from build123d import *

# Parameters (mm, degrees)
F0_W          = 76.2
F0_H          = 38.1
F1_DEPTH      = 12.7
F2_R          = 19.05
F3_DEPTH      = 19.05
F4_R          = 19.05
F5_DEPTH      = 19.05
F6_R          = 7.9375
F7_DEPTH      = 19.051
F7_DEPTH_BACK = 31.751
F9_START      = -6.35
F8_R          = 14.9225
F8_R_2        = 7.9375
F9_DEPTH      = 6.35


with BuildPart() as f1:
    # F0 (on Top) → F1 (new body)
    with BuildSketch(Plane.XY):
        with Locations((38.1, 19.05)):
            Rectangle(F0_W, F0_H)
    extrude(amount=F1_DEPTH)

    # F2 (on face) → F3 (join)
    with BuildSketch(Plane.XY.offset(12.7)):
        with Locations((38.1, 19.05)):
            Circle(F2_R)
    extrude(amount=F3_DEPTH)

    # F4 (on face) → F5 (join)
    with BuildSketch(Plane(origin=(0, 0, 0), x_dir=(1, 0, 0), z_dir=(0, 0, -1))):
        with Locations((38.1, -19.05)):
            Circle(F4_R)
    extrude(amount=F5_DEPTH)

    # F6 (on Top) → F7 (cut, two sides)
    with BuildSketch(Plane.XY) as f7_sk:
        with Locations((38.1, 19.05)):
            Circle(F6_R)
    extrude(amount=-F7_DEPTH, mode=Mode.SUBTRACT)
    extrude(f7_sk.sketch, amount=F7_DEPTH_BACK, mode=Mode.SUBTRACT)

    # F8 (on face) → F9 (cut)
    with BuildSketch(Plane.XY.offset(31.75).offset(F9_START)):
        with Locations((38.1, 19.05)):
            Circle(F8_R)
        with Locations((38.1, 19.05)):
            Circle(F8_R_2, mode=Mode.SUBTRACT)
    extrude(amount=-F9_DEPTH, mode=Mode.SUBTRACT)


solid = f1.part
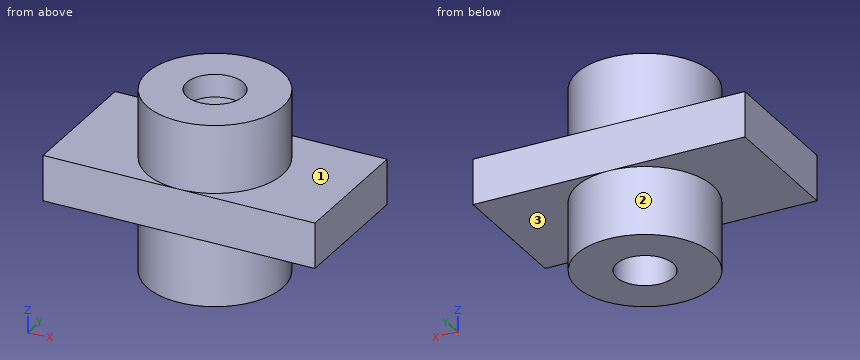
Part model, mm, in its own coordinate system. Face numbers are marked on the shaded views. A direction names the side the tool comes from. Coordinates: 2 decimals unless noted, no trailing zeros. Order: outer loops, then holes, each group sorted by start corner. A loop starts at its lowest first (then second) coordinate and runs counter-clockwise, first axis right, second up. Notation, with made-up numbers: (-0.75, 4.5) - (44.25, 4.5) arc R22 cw to (44.25, 22.5) - close; hole circle Ø8 at (88, 8.25). An arc over 180 degrees is marked (long way). Use CSV: the item, a comma, the result in double quotes.
Item 1: Saw through at A-A on y = 19.05. Give the cut face in (x, z).
Solved:
outline,"(0, 0) - (19.05, 0) - (19.05, -19.05) - (30.16, -19.05) - (30.16, 19.05) - (23.18, 19.05) - (23.18, 25.4) - (30.16, 25.4) - (30.16, 31.75) - (19.05, 31.75) - (19.05, 12.7) - (0, 12.7) - close; (46.04, -19.05) - (57.15, -19.05) - (57.15, 0) - (76.2, 0) - (76.2, 12.7) - (57.15, 12.7) - (57.15, 31.75) - (46.04, 31.75) - (46.04, 25.4) - (53.02, 25.4) - (53.02, 19.05) - (46.04, 19.05) - close"
Item 2: Saw through at C-C on x = 49. Give the cut face in (y, z), and give its area (3 significant figures).
Solved:
outline,"(0, 0) - (3.43, 0) - (3.43, -19.05) - (34.67, -19.05) - (34.67, 0) - (38.1, 0) - (38.1, 12.7) - (34.67, 12.7) - (34.67, 31.75) - (3.43, 31.75) - (3.43, 12.7) - (0, 12.7) - close; hole (8.86, 19.05) - (29.24, 19.05) - (29.24, 25.4) - (8.86, 25.4) - close"
area,"1,540 mm²"
Item 3: Probe probe 1 along Y at (x, z) = (38, 16.5); probe 2 along Y at (x, z) = (38.1, 21.25); probe 3 along Z at (x, y) = (50.5, 26.5). List the from-to ranges inside material, lowest first.
Solved:
probe 1,"y = 0 to 11.11, 26.99 to 38.1"
probe 2,"y = 0 to 4.13, 33.97 to 38.1"
probe 3,"z = -19.05 to 19.05, 25.4 to 31.75"
Item 4: Saw through at B-B on x = 36. Give the cut face in (y, z), and give its area (3 significant figures).
Solved:
outline,"(0, 0) - (0.12, 0) - (0.12, -19.05) - (11.4, -19.05) - (11.4, 19.05) - (4.28, 19.05) - (4.28, 25.4) - (11.4, 25.4) - (11.4, 31.75) - (0.12, 31.75) - (0.12, 12.7) - (0, 12.7) - close; (26.7, -19.05) - (37.98, -19.05) - (37.98, 0) - (38.1, 0) - (38.1, 12.7) - (37.98, 12.7) - (37.98, 31.75) - (26.7, 31.75) - (26.7, 25.4) - (33.82, 25.4) - (33.82, 19.05) - (26.7, 19.05) - close"
area,"1,060 mm²"
Item 5: Drop flat-ended pins along their axis: P1, Ø6, axis at y = 9.5, z = 15.5, coming from the -X side; P2, Ø1, axis at y = 28.5, z = -12.5, coming from the -X side; P3, Ø8, axis at y = 11, z = 21.5, coming from the +X side; P4, Ø3, axis at x = 63.5, y = 32, coming from the -Z side. Give the stop position or say it passes through.
Solved:
P1,"stops at x = 0"
P2,"stops at x = 21.28"
P3,"stops at x = 56.71"
P4,"stops at z = 0"
Item 6: 3-axis set-ups, long thin cutter, end or side, ignore diameter. For the marked faces 1, 2 and 3: which of +Z, -Z, +X, -X, +Y, -Y reach the whole face in a straight line?
Solved:
face 1,"+Z, +X"
face 2,"-Z"
face 3,"-Z, +X"
